```python
from build123d import *

# Parameters (mm, degrees)
SKETCH1_W           = 26
SKETCH1_H           = 36
BOSS_EXTRUDE1_DEPTH = 7
BOSS_EXTRUDE1_DRAFT = -1
FILLET1_R           = 6
SHELL1_T            = -3
EXTRUDE_THIN1_DEPTH = 2


# Read off the part's stored shape, not the designer's step: Extrude-Thin1
with BuildPart() as part:
    # Sketch1 → Boss-Extrude1 (with draft: the straight prism first)
    with BuildSketch(Plane(origin=(0, 0, 0), x_dir=(1, 0, 0), z_dir=(0, 1, 0))):
        Rectangle(SKETCH1_W, SKETCH1_H)
    extrude(amount=BOSS_EXTRUDE1_DEPTH)
    # Boss-Extrude1: the draft: its side faces are tilted about the plane it starts from
    boss_extrude1_sides = [part.faces().sort_by_distance(p)[0] for p in [
        (-13, 3.5, 0),
        (0, 3.5, 18),
        (13, 3.5, 0),
        (0, 3.5, -18),
    ]]
    draft(boss_extrude1_sides, Plane(origin=(0, 0, 0), x_dir=(1, 0, 0), z_dir=(0, 1, 0)), BOSS_EXTRUDE1_DRAFT)

    # Fillet1
    fillet1_edges = [part.edges().sort_by_distance(p)[0] for p in [
        (0, 0, 18),
        (-13, 0, 0),
        (0, 0, -18),
        (13, 0, 0),
        (13.061092727, 3.5, 18.061092727),
        (-13.061092727, 3.5, 18.061092727),
        (-13.061092727, 3.5, -18.061092727),
        (13.061092727, 3.5, -18.061092727),
    ]]
    fillet(fillet1_edges, radius=FILLET1_R)

    # Shell1
    shell1_openings = [part.faces().sort_by_distance(p)[0] for p in [
        (0, 7, 0),
    ]]
    offset(amount=SHELL1_T, openings=shell1_openings, kind=Kind.INTERSECTION)

    # Extrude-Thin1 outline → Extrude-Thin1 (add)
    with BuildSketch(Plane(origin=(0, 7, 0), x_dir=(1, 0, 0), z_dir=(0, 1, 0))):
        with BuildLine():
            Line((-11.503359551, 12.103816421), (-11.503359551, -12.103816421))
            add(Edge.make_bspline(
                [(-11.503359551, -12.103816421), (-11.503239974, -12.679639127), (-11.388644012, -13.255211042), (-10.94780799, -14.319148914), (-10.621742234, -14.807098768), (-9.807439748, -15.62148016), (-9.319521491, -15.947593193), (-8.261151516, -16.386242364), (-7.692017173, -16.500790934), (-7.122185385, -16.503316936)],
                knots=[0, 0, 0, 0, 0.25, 0.25, 0.5, 0.5, 0.75, 0.75, 0.997403327, 0.997403327, 0.997403327, 0.997403327], degree=3))
            Line((-7.122185385, -16.503316936), (-7.122185385, -16.52172847))
            Line((-7.122185385, -16.52172847), (7.122185385, -16.52172847))
            add(Edge.make_bspline(
                [(7.122185385, -16.52172847), (7.698092154, -16.52172847), (8.273773075, -16.407240069), (9.337918721, -15.966495827), (9.825962781, -15.640412314), (10.640412314, -14.825962781), (10.966495827, -14.337918721), (11.407240069, -13.273773075), (11.52172847, -12.698092154), (11.52172847, -12.122185385)],
                knots=[0, 0, 0, 0, 0.25, 0.25, 0.5, 0.5, 0.75, 0.75, 1, 1, 1, 1], degree=3))
            Line((11.52172847, -12.122185385), (11.52172847, 12.122185385))
            add(Edge.make_bspline(
                [(11.52172847, 12.122185385), (11.52172847, 12.698092154), (11.407240069, 13.273773075), (10.966495827, 14.337918721), (10.640412314, 14.825962781), (9.825962781, 15.640412314), (9.337918721, 15.966495827), (8.273773075, 16.407240069), (7.698092154, 16.52172847), (7.122185385, 16.52172847)],
                knots=[0, 0, 0, 0, 0.25, 0.25, 0.5, 0.5, 0.75, 0.75, 1, 1, 1, 1], degree=3))
            Line((7.122185385, 16.52172847), (7.122185385, 15.12172847))
            add(Edge.make_bspline(
                [(10.12172847, 12.122185385), (10.12172847, 15.12172847), (7.122185385, 15.12172847)],
                knots=[2.356346783, 2.356346783, 2.356346783, 3.926838524, 3.926838524, 3.926838524], degree=2, weights=[1, 0.707214461, 1]))
            Line((10.12172847, 12.122185385), (10.12172847, -12.122185385))
            add(Edge.make_bspline(
                [(7.122185385, -15.12172847), (10.12172847, -15.12172847), (10.12172847, -12.122185385)],
                knots=[2.356346783, 2.356346783, 2.356346783, 3.926838524, 3.926838524, 3.926838524], degree=2, weights=[1, 0.707214461, 1]))
            Line((7.122185385, -15.12172847), (-7.103822016, -15.12172847))
            Line((-7.103822016, -15.12172847), (-7.103816421, -15.103359507))
            add(Edge.make_bspline(
                [(-10.103359507, -12.103816421), (-10.102446165, -15.102446165), (-7.103816421, -15.103359507)],
                knots=[3.92714311, 3.92714311, 3.92714311, 5.497634851, 5.497634851, 5.497634851], degree=2, weights=[1, 0.707214461, 1]))
            Line((-10.103359507, -12.103816421), (-10.103359507, 12.103816421))
            add(Edge.make_bspline(
                [(-7.103816421, 15.103359507), (-10.102446165, 15.102446165), (-10.103359507, 12.103816421)],
                knots=[3.92714311, 3.92714311, 3.92714311, 5.497634851, 5.497634851, 5.497634851], degree=2, weights=[1, 0.707214461, 1]))
            Line((-7.103816421, 15.103359507), (7.103816421, 15.103359507))
            Line((7.103816421, 15.103359507), (7.103816421, 16.503359507))
            Line((7.103816421, 16.503359507), (-7.103816421, 16.503359551))
            add(Edge.make_bspline(
                [(-7.103816421, 16.503359551), (-7.679674662, 16.503239967), (-8.255282039, 16.388629695), (-9.319274889, 15.947740691), (-9.807244134, 15.621636328), (-10.621636328, 14.807244134), (-10.947740691, 14.319274889), (-11.388629695, 13.255282039), (-11.503239967, 12.679674662), (-11.503359551, 12.103816421)],
                knots=[0, 0, 0, 0, 0.25, 0.25, 0.5, 0.5, 0.75, 0.75, 1, 1, 1, 1], degree=3))
        make_face()
    extrude(amount=EXTRUDE_THIN1_DEPTH)


solid = part.part
```
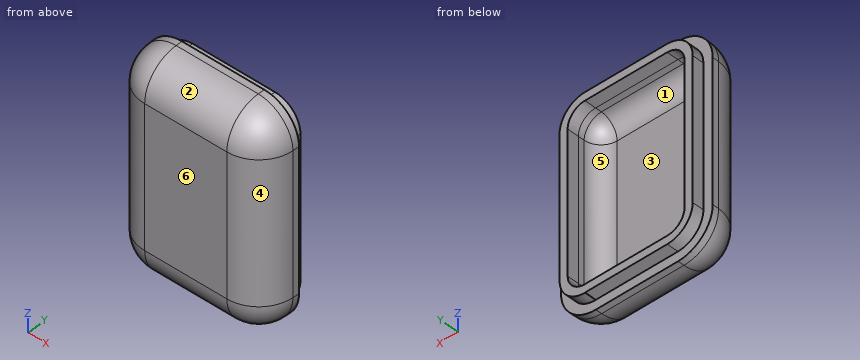
Read the model definition and answer for the solid it produces. Units are mm, in the model's axes. Face numbers are marked on the shaded views. A direction names the side the tool comes from. Give positions to 0.01 mm unless a question says otherwise; leave off trailing zeros. Loops run counter-clockwise (first coordinate to the right, second up) from the corner with the lowest first, then second, coordinate; pieces in that order, holes last.
Item 1: For the marked faces 5 and 6, determine the directions among +Z, -Z, +X, -X, +Y, -Y from which every point of the face is accessible in a straight line to the end or side of a thin tool.
Item 2: The mould has two halves that part along Z. Classify the marked faces 1, 2, 3 and 4: released by +Z, released by -Z, zero draft, split by the parting line, or undercut.
Item 3: Find the intervals of material crossed by line 1 along X through (y, z) = (6.5, 0); line 2 along Z through (x, y) = (-3.25, 7.5); line 3 along X through (y, z) = (7.25, -11), in increasing order.
Item 4: Each of these flat-tipped pins is pushed along its axis until it touches: pin 1 Ø6 at (x, z) = (1.5, 1) entering from +Y; pin 2 Ø1.5 at (y, z) = (2, -8.5) entering from +X; pin 3 Ø1 at (x, y) = (1, 8) entering from -Z. Where does it stop, or does it pass through?
Item 5: The part is cut by section A-A (y = 4.5). Write down the section's boundary in (x, z).
Item 6: The part is cut by section D-D (y = 1). Write down the section's boundary in (x, z), and give its area (3 significant figures).
Taken from the geometry:
1. face 5: +Y
1. face 6: +Z, -Z, +X, -X, -Y
2. face 1: undercut
2. face 2: released by +Z
2. face 3: undercut
2. face 4: zero draft
3. line 1: x = -13.11 to -10.11, 10.11 to 13.11
3. line 2: z = -16.5 to -15.1, 15.12 to 16.52
3. line 3: x = -11.5 to -10.1, 10.12 to 11.52
4. pin 1: stops at y = 3
4. pin 2: stops at x = 12.15
4. pin 3: stops at z = -16.5
5. outline: (-12.91, -12.1) arc R5.81 ccw to (-7.1, -17.91) - (7.1, -17.91) arc R5.81 ccw to (12.91, -12.1) - (12.91, 12.1) arc R5.81 ccw to (7.1, 17.91) - (-7.1, 17.91) arc R5.81 ccw to (-12.91, 12.1) - close; hole (-9.7, -12.1) arc R2.6 ccw to (-7.1, -14.7) - (7.1, -14.7) arc R2.6 ccw to (9.7, -12.1) - (9.7, 12.1) arc R2.6 ccw to (7.1, 14.7) - (-7.1, 14.7) arc R2.6 ccw to (-9.7, 12.1) - close
6. outline: (-10.42, -12.1) arc R3.32 ccw to (-7.1, -15.42) - (7.1, -15.42) arc R3.32 ccw to (10.42, -12.1) - (10.42, 12.1) arc R3.32 ccw to (7.1, 15.42) - (-7.1, 15.42) arc R3.32 ccw to (-10.42, 12.1) - close
6. area: 633 mm2
